from build123d import *

# Parameters (mm, degrees)
F0_W     = 220
F0_H     = 150
F0_R     = 61.5
F2_DEPTH = 10
F1_W     = 20
F1_H     = 41
F1_R     = 2.19
F3_DEPTH = 10


with BuildPart() as f2:
    # F0 (on Top) → F2 (new body)
    with BuildSketch(Plane.XY):
        Rectangle(F0_W, F0_H)
        with Locations((0, -5.5)):
            Circle(F0_R, mode=Mode.SUBTRACT)
    extrude(amount=-F2_DEPTH)

    # F1 (on Top) → F3 (cut, through all)
    with BuildSketch(Plane.XY):
        with Locations((-85.3, -16.18)):
            Rectangle(F1_W, F1_H)
        with Locations((-80.375, 7.97)):
            Circle(F1_R)
        with Locations((-90.225, 7.97)):
            Circle(F1_R)
        with Locations((-80.375, -40.33)):
            Circle(F1_R)
        with Locations((-90.225, -40.33)):
            Circle(F1_R)
        with Locations((85.3, -16.18)):
            Rectangle(F1_W, F1_H)
        with Locations((80.375, 7.97)):
            Circle(F1_R)
        with Locations((90.225, 7.97)):
            Circle(F1_R)
        with Locations((80.375, -40.33)):
            Circle(F1_R)
        with Locations((90.225, -40.33)):
            Circle(F1_R)
    extrude(amount=-F3_DEPTH, mode=Mode.SUBTRACT)


solid = f2.part
Geometry check sheet. Reference: the model listing, model coordinates, mm. A direction names the side the tool comes from. Coordinates: 2 decimals unless noted, no trailing zeros. Order: outer loops, then holes, each group sorted by start corner. A loop starts at its lowest first (then second) coordinate and runs counter-clockwise, first axis right, second up. Notation, with made-up numbers: (87.5, 84.25) - (123.5, 84.25) arc R18 ccw to (123.5, 104.25) - close; hole circle Ø2 at (48.25, -5.75). An arc over 180 degrees is marked (long way). Answer in a Markdown table with one row per item. Add a question column.
1) Release check for a two-part mould opening along Y. For faces 3 (the flat face through (-2, 75, -5)), 4 (the flat face through (-110, -1, -5)), 5 (the flat face through (85, 4.32, -5)) record: +Y half, -Y half, draft (parallel to the pull), parting line (faces both ways), or undercut.
2) Cross-section at B-B, the plane x = 5.5. Record the cut outline in (y, z).
3) Cross-section at A-A, the plane y = -5.5. Record the cut outline in (x, z), then the cut area to 3 significant figures.
4) Set-up check for faces 1 (the flat face through (-26, 51, -10)), 2 (the flat face through (75.3, -16, -5)): record each of +Z, -Z, +X, -X, +Y, -Y from which the full face is reachable in a straight line by a thin tool's end or side.
5) Cross-section at D-D, the plane y = 17. Record the cut outline in (x, z), then the cut area to 3 significant figures.
6) Cross-section at C-C, the plane z = -3.75. State how many separate pieces and enclosed holes the cut face has, then the cut area to 3 significant figures.
7) Gauge pin test, flat end, axial feed: P1, Ø5, axis at x = 90.225, y = -40.33, coming from the -Z side. Record the tip position at first contact, or that the pin passes through.
8) Material ranges on line 1 along Y through (x, z) = (0, -5.5); line 2 along Y through (x, z) = (95, -5); line 3 along X through (y, z) = (-33.5, -6.75), recorded low to high. Write a range as [from, to].
Check result:
| question | item | result |
|---|---|---|
| 1 | face 3 | +Y half |
| 1 | face 4 | draft |
| 1 | face 5 | undercut |
| 2 | outline | (-75, -10) - (-66.75, -10) - (-66.75, 0) - (-75, 0) - close; (55.75, -10) - (75, -10) - (75, 0) - (55.75, 0) - close |
| 3 | outline | (-110, -10) - (-95.3, -10) - (-95.3, 0) - (-110, 0) - close; (-75.3, -10) - (-61.5, -10) - (-61.5, 0) - (-75.3, 0) - close; (61.5, -10) - (75.3, -10) - (75.3, 0) - (61.5, 0) - close; (95.3, -10) - (110, -10) - (110, 0) - (95.3, 0) - close |
| 3 | area | 570 mm² |
| 4 | face 1 | -Z, +X, -X, +Y, -Y |
| 4 | face 2 | +Z, -Z |
| 5 | outline | (-110, -10) - (-57.24, -10) - (-57.24, 0) - (-110, 0) - close; (57.24, -10) - (110, -10) - (110, 0) - (57.24, 0) - close |
| 5 | area | 1,060 mm² |
| 6 | separate pieces | 1 |
| 6 | enclosed holes | 11 |
| 6 | area | 19,400 mm² |
| 7 | P1 | stops at z = -10 |
| 8 | line 1 | y = [-75, -67], [56, 75] |
| 8 | line 2 | y = [-75, -36.68], [4.32, 75] |
| 8 | line 3 | x = [-110, -95.3], [-75.3, -54.76], [54.76, 75.3], [95.3, 110] |
